Source: three-view drawing plus pictorial views. Frame: mm from the lowest corner of the part. A direction names the side the tool comes from. Round coordinates to 2 decimals unless told otherwise and drop trailing zeros. Write each loop counter-clockwise with the first axis right and the second up, starting at its lowest first coordinate (ties: lowest second). Pieces come first, ordered by that corner, then holes. Notation, with made-up numbers: M 30.25,23 L 86.25,23 A15 ccw 86.25,49 Z; hole C -15.75,50 d2. An arc over 180 degrees is marked long. Answer in a Markdown table with one row per item.
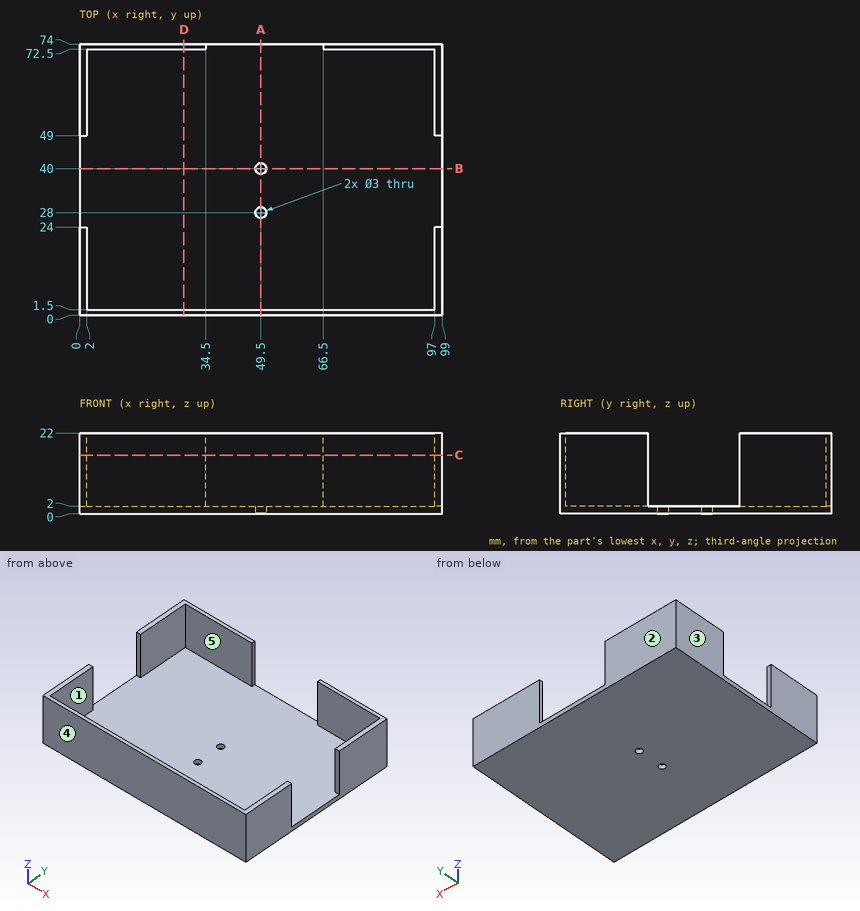
Q1. Section C-C (z = 16). Return loops of the section in (x, y), and give its area (3 significant figures).
Solutions:
| item | result |
|---|---|
| outline | M 0,0 L 99,0 L 99,24 L 97,24 L 97,1.5 L 2,1.5 L 2,24 L 0,24 Z; M 0,49 L 2,49 L 2,72.5 L 34.5,72.5 L 34.5,74 L 0,74 Z; M 66.5,72.5 L 97,72.5 L 97,49 L 99,49 L 99,74 L 66.5,74 Z |
| area | 433 mm2 |
Q2. Pull-direction query (Y, two-part tool) for the marked faces 3, 4 and 5; classes: pulls with the +Y half, pulls with the -Y half, needs draft (parallel to the pull), parting line crosses it, or undercut.
Solutions:
| item | result |
|---|---|
| face 3 | needs draft |
| face 4 | pulls with the -Y half |
| face 5 | undercut |
Q3. Section A-A (x = 49.5). Return loops of the section in (y, z), and give its area (3 significant figures).
Solutions:
| item | result |
|---|---|
| outline | M 0,0 L 26.5,0 L 26.5,2 L 1.5,2 L 1.5,22 L 0,22 Z; M 29.5,0 L 38.5,0 L 38.5,2 L 29.5,2 Z; M 41.5,0 L 74,0 L 74,2 L 41.5,2 Z |
| area | 166 mm2 |
Q4. Access query for the marked faces 1 and 2. Directions: +Z, -Z, +X, -X, +Y, -Y. A direction counts if a zero-diameter tool reaches every point of the face in a straight line with its end or side. Return the directions, or none.
Solutions:
| item | result |
|---|---|
| face 1 | +Z |
| face 2 | +Z, -Z, +X, -X, +Y |
Q5. Section B-B (y = 40). Return loops of the section in (x, z), and give its area (3 significant figures).
Solutions:
| item | result |
|---|---|
| outline | M 0,0 L 48,0 L 48,2 L 0,2 Z; M 51,0 L 99,0 L 99,2 L 51,2 Z |
| area | 192 mm2 |
Q6. Contact query for a flat-ended pin moving along its axis: pin 1 Ø8 at (x, y) = (10.5, 39) entering from +Z. Output: stop coordinate, or through.
Solutions:
| item | result |
|---|---|
| pin 1 | stops at z = 2 |
Q7. Material intervals for probe 1 along Y at (x, z) = (49.5, 1.15); probe 2 along X at (y, z) = (70.5, 12); probe 3 along Y at (x, z) = (4.5, 14.75), sorted ascending.
Solutions:
| item | result |
|---|---|
| probe 1 | y = 0 to 26.5, 29.5 to 38.5, 41.5 to 74 |
| probe 2 | x = 0 to 2, 97 to 99 |
| probe 3 | y = 0 to 1.5, 72.5 to 74 |
Q8. Section D-D (x = 28.5). Return loops of the section in (y, z).
Solutions:
| item | result |
|---|---|
| outline | M 0,0 L 74,0 L 74,22 L 72.5,22 L 72.5,2 L 1.5,2 L 1.5,22 L 0,22 Z |
